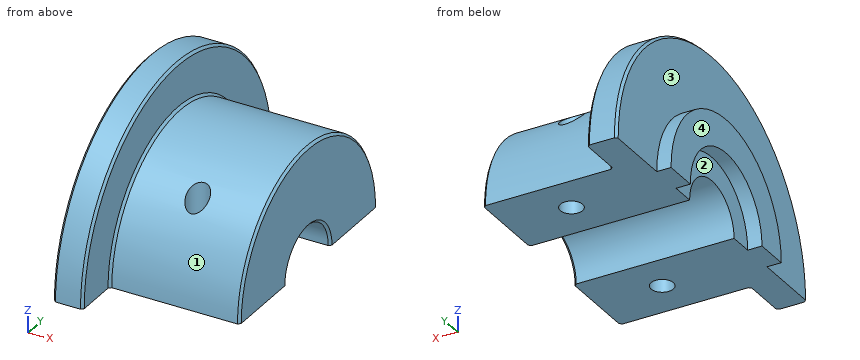
```python
from build123d import *

# Parameters (mm, degrees)
SKETCH1_R           = 12.6365
BOSS_EXTRUDE1_DEPTH = 21.844
SKETCH2_R           = 17.526
BOSS_EXTRUDE2_DEPTH = 3.175
CHAMFER1_SIZE       = 0.254
SKETCH3_R           = 4.09575
CUT_EXTRUDE1_DEPTH  = 34.037579936
CHAMFER2_SIZE       = 0.254
SKETCH4_R           = 1.984375
CUT_EXTRUDE2_DEPTH  = 22.606
SKETCH5_R           = 12.8905
CUT_EXTRUDE3_DEPTH  = 4.7625
SKETCH6_W           = 26.198256486
SKETCH6_H           = 39.009491802
CUT_EXTRUDE4_DEPTH  = 41.783
SKETCH7_R           = 1.190625
CUT_EXTRUDE5_DEPTH  = 12.7
BOSS_EXTRUDE3_DEPTH = 1.524


with BuildPart() as part:
    # Sketch1 → Boss-Extrude1 (new body)
    with BuildSketch(Plane(origin=(0, 0, 0), x_dir=(0, 0, -1), z_dir=(1, 0, 0))):
        Circle(SKETCH1_R)
    extrude(amount=BOSS_EXTRUDE1_DEPTH)

    # Sketch2 → Boss-Extrude2 (add)
    with BuildSketch(Plane(origin=(7.9375, 0, 0), x_dir=(0, 0, -1), z_dir=(1, 0, 0))):
        Circle(SKETCH2_R)
    extrude(amount=-BOSS_EXTRUDE2_DEPTH)

    # Chamfer1
    chamfer1_edges = [part.edges().sort_by_distance(p)[0] for p in [
        (0, 0, 12.6365),
        (21.844, 0, 12.6365),
        (4.7625, 0, 12.6365),
        (7.9375, 0, 12.6365),
        (4.7625, 0, 17.526),
        (7.9375, 0, 17.526),
    ]]
    chamfer(chamfer1_edges, length=CHAMFER1_SIZE)

    # Sketch3 → Cut-Extrude1 (cut, through all)
    with BuildSketch(Plane(origin=(21.844, 0, 0), x_dir=(0, 0, -1), z_dir=(1, 0, 0))):
        Circle(SKETCH3_R)
    extrude(amount=-CUT_EXTRUDE1_DEPTH, mode=Mode.SUBTRACT)

    # Chamfer2
    chamfer2_edges = [part.edges().sort_by_distance(p)[0] for p in [
        (0, 0, 4.09575),
        (21.844, 0, 4.09575),
    ]]
    chamfer(chamfer2_edges, length=CHAMFER2_SIZE)

    # Sketch4 → Cut-Extrude2 (cut)
    with BuildSketch(Plane.XY):
        with Locations((14.89075, 0)):
            Circle(SKETCH4_R)
    extrude(amount=-CUT_EXTRUDE2_DEPTH, mode=Mode.SUBTRACT)

    # Sketch5 → Cut-Extrude3 (cut)
    with BuildSketch(Plane.ZY):
        Circle(SKETCH5_R)
    extrude(amount=-CUT_EXTRUDE3_DEPTH, mode=Mode.SUBTRACT)

    # Sketch6 → Cut-Extrude4 (cut)
    with BuildSketch(Plane.XY):
        with Locations((13.991232321, 0)):
            Rectangle(SKETCH6_W, SKETCH6_H)
    extrude(amount=-CUT_EXTRUDE4_DEPTH, mode=Mode.SUBTRACT)

    # Sketch7 → Cut-Extrude5 (cut)
    with BuildSketch(Plane(origin=(0, 0, 0), x_dir=(-1, 0, 0), z_dir=(0, 0, -1))):
        with Locations((-14.89075, 8.366125)):
            Circle(SKETCH7_R)
    cut_extrude5 = extrude(amount=-CUT_EXTRUDE5_DEPTH, mode=Mode.SUBTRACT)

    # Mirror1: Cut-Extrude5 across plane
    add(cut_extrude5.mirror(Plane.ZX), mode=Mode.SUBTRACT)

    # Sketch8 → Boss-Extrude3 (add)
    with BuildSketch(Plane.ZY.offset(-4.7625)):
        with BuildLine():
            Line((0, -10.16), (0, -6.604))
            ThreePointArc((0, -6.604), (6.604, 0), (0, 6.604))
            Line((0, 6.604), (0, 10.16))
            ThreePointArc((0, 10.16), (10.16, 0), (0, -10.16))
        make_face()
    extrude(amount=BOSS_EXTRUDE3_DEPTH)


solid = part.part
```
Geometry check sheet. Reference: the model listing, model coordinates, mm. Face numbers are marked on the shaded views. A direction names the side the tool comes from. Round coordinates to 2 decimals unless told otherwise and drop trailing zeros. Order: outer loops, then holes, each group sorted by start corner. A loop starts at its lowest first (then second) coordinate and runs counter-clockwise, first axis right, second up. Notation, with made-up numbers: (-14.75, 44.5) - (-4.75, 44.5) arc R23 cw to (-4.75, 58.5) - close; hole circle Ø8 at (81.5, 78.5). An arc over 180 degrees is marked (long way). Use a Markdown table: item, result. Add a question column.
1) Section check C-C (x = 7.25). Record the cut outline in (y, z).
2) Section check D-D (z = 7.25). Count the separate pieces of the cut face and the enclosed holes in it, then the cut area to 3 significant figures.
3) Thickness scan on line 1 along Y through (x, z) = (14.25, 4.5); line 2 along Y through (x, z) = (14, 3.75); line 3 along Y through (x, z) = (10, 3.75). Record the ranges inside material, lowest first.
4) Section check A-A (x = 14.25). Record the cut outline in (y, z), then the cut area to 3 significant figures.
5) Set-up check for the marked faces 1, 2, 3 and 4: record each of +Z, -Z, +X, -X, +Y, -Y from which the full face is reachable in a straight line by a thin tool's end or side.
6) Gauge pin test, flat ends, axial feed: P1, Ø3, axis at y = 8, z = 12.5, coming from the +X side; P2, Ø1.9, axis at x = 14.89, y = -8.37, coming from the -Z side; P3, Ø4, axis at x = 8.5, z = 7, coming from the +Y side; P4, Ø3, axis at x = 8.5, y = 2.5, coming from the +Z side. Record the tip position at first contact, or that the pin passes through.
7) Section check B-B (y = 0). Record the cut outline in (x, z), then the cut area to 3 significant figures.
Established:
| question | item | result |
|---|---|---|
| 1 | outline | (-17.53, 0) - (-4.1, 0) arc R4.1 cw to (4.1, 0) - (17.53, 0) arc R17.53 ccw to start |
| 2 | separate pieces | 1 |
| 2 | enclosed holes | 2 |
| 2 | area | 402 mm2 |
| 3 | line 1 | -11.81 to -9.37, -7.36 to 7.36, 9.37 to 11.81 |
| 3 | line 2 | -12.07 to -9.16, -7.58 to -1.65, 1.65 to 7.58, 9.16 to 12.07 |
| 3 | line 3 | -12.07 to -1.65, 1.65 to 12.07 |
| 4 | outline | (-12.64, 0) - (-9.37, 0) - (-9.37, 8.48) arc R12.64 ccw to start; (-7.36, 0) - (-4.1, 0) arc R4.1 cw to (4.1, 0) - (7.36, 0) - (7.36, 10.27) arc R12.64 ccw to (-7.36, 10.27) - close; (9.37, 0) - (12.64, 0) arc R12.64 ccw to (9.37, 8.48) - close |
| 4 | area | 187 mm2 |
| 5 | face 1 | +Z, +X |
| 5 | face 2 | -Z, -X |
| 5 | face 3 | +Z, -X |
| 5 | face 4 | +Z, -Z, -X, +Y, -Y |
| 6 | P1 | x = 7.94 |
| 6 | P2 | through |
| 6 | P3 | y = 16.74 |
| 6 | P4 | z = 17.48 |
| 7 | outline | (3.24, 6.6) - (4.76, 6.6) - (4.76, 4.1) - (21.59, 4.1) - (21.84, 4.35) - (21.84, 12.38) - (21.59, 12.64) - (8.19, 12.64) - (7.94, 12.89) - (7.94, 17.27) - (7.68, 17.53) - (5.02, 17.53) - (4.76, 17.27) - (4.76, 10.16) - (3.24, 10.16) - close |
| 7 | area | 167 mm2 |
